Can you work these out from the model? Positions are in its coordinate system, mm. Coordinates: 2 decimals unless noted, no trailing zeros. Order: outer loops, then holes, each group sorted by start corner. A loop starts at its lowest first (then second) coordinate and runs counter-clockwise, first axis right, second up. Notation, with made-up numbers: (-6, 60) -> (31, 60) arc R19 cw to (31, 90) -> close; hole circle Ø1 at (73.5, -4.75). An arc over 180 degrees is marked (long way). Return JSON: item names as keys, results as strings. Group by question number.
1) For pin 1 (3 mm diameter, centred on x = 2.5, z = -5, fed in from -Y); pin 2 (0.8 mm diameter, centred on x = 34, y = 1, fed in from -Z); pin 3 (0.8 mm diameter, centred on y = 1, z = -43, fed in from +X), each with a flat end and sliding along its axis, tell me the tip position at first contact or that it passes through.
2) If we section it at C-C, the plane z = -42.5: Please give me the cut outline in (x, y), then the cut area to 3 significant figures.
3) If I drill on probe 1 along X at (y, z) = (1, -53.5); probe 2 along X at (y, z) = (1.05, -40), over which ranges is the centre line in solid material (lowest first)? Write a range as from..to.
4) If we section it at B-B, the plane z = -61.5: Please give me the cut outline in (x, y).
5) If we section it at A-A, the plane y = 0.45: Please give me the cut outline in (x, z).
from build123d import *

# Parameters (mm, degrees)
FR4_DEPTH = 1.5875


with BuildPart() as part:
    # Sketch1 → FR4 (new body)
    with BuildSketch(Plane(origin=(0, 0, 0), x_dir=(1, 0, 0), z_dir=(0, 1, 0))):
        with BuildLine():
            Line((34.5, -9), (34.5, 36))
            Line((34.5, 36), (32.940007652, 36))
            ThreePointArc((32.940007652, 36), (32.271894631, 36.313775841), (32, 37))
            Line((32, 37), (32, 46.75))
            Line((32, 46.75), (31, 46.75))
            ThreePointArc((31, 46.75), (30.292893219, 47.042893219), (30, 47.75))
            Line((30, 47.75), (30, 67.5))
            Line((30, 67.5), (-31.3, 67.5))
            Line((-31.3, 67.5), (-31.3, 41.5))
            ThreePointArc((-31.3, 41.5), (-31.564481186, 40.821086647), (-32.218527823, 40.5))
            Line((-32.218527823, 40.5), (-34.5, 40.5))
            Line((-34.5, 40.5), (-34.5, -9))
            Line((-34.5, -9), (-34.5, -16))
            Line((-34.5, -16), (34.5, -16))
            Line((34.5, -16), (34.5, -9))
        make_face()
    extrude(amount=FR4_DEPTH)


solid = part.part
Result sheet:
{
 "1": {"pin 1": "stops at y = 0", "pin 2": "stops at z = -36", "pin 3": "stops at x = 32"},
 "2": {"outline": "(-31.3, 0) -> (32, 0) -> (32, 1.59) -> (-31.3, 1.59) -> close", "area": "100 mm2"},
 "3": {"probe 1": "x = -31.3..30", "probe 2": "x = -34.5..32"},
 "4": {"outline": "(-31.3, 0) -> (30, 0) -> (30, 1.59) -> (-31.3, 1.59) -> close"},
 "5": {"outline": "(-34.5, -40.5) -> (-32.22, -40.5) arc R1 cw to (-31.3, -41.5) -> (-31.3, -67.5) -> (30, -67.5) -> (30, -47.75) arc R1 cw to (31, -46.75) -> (32, -46.75) -> (32, -37) arc R1 cw to (32.94, -36) -> (34.5, -36) -> (34.5, 16) -> (-34.5, 16) -> close"}
}
